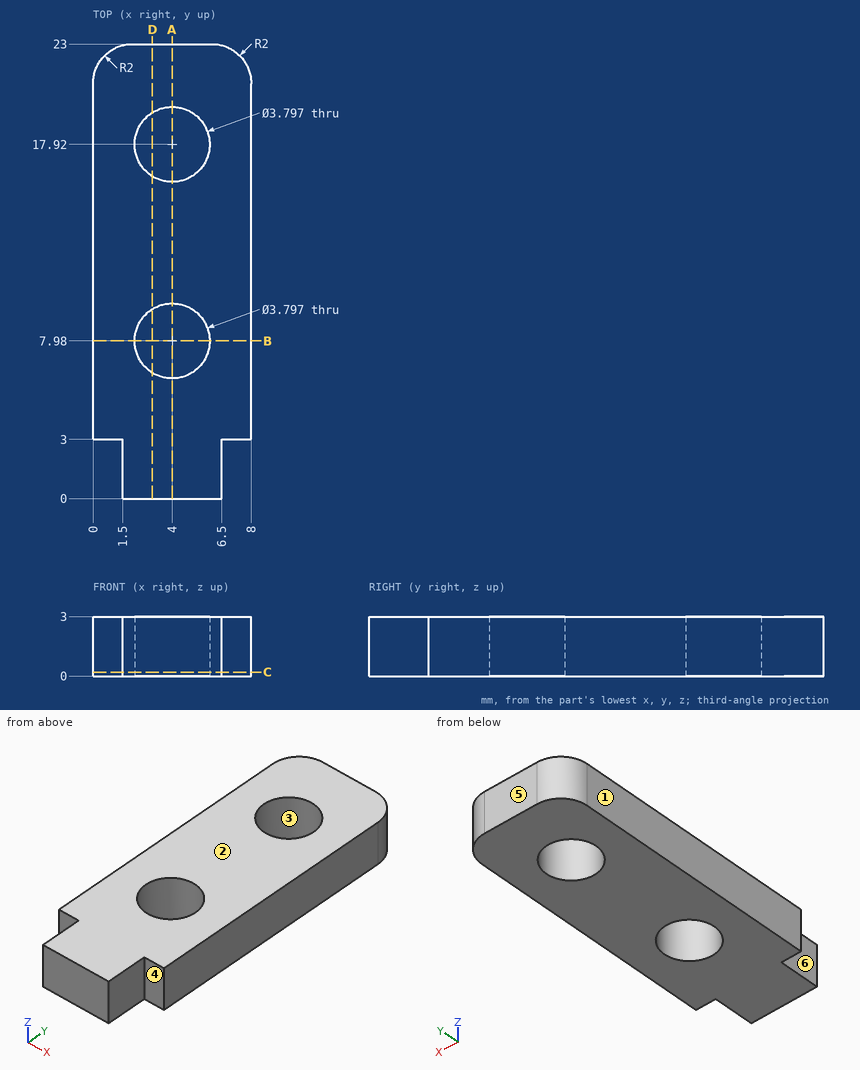
Here's the drawing with two shaded views (mm, measured from the low corner). I have some questions. A direction names the side the tool comes from. Give positions to 0.01 mm unless a question says otherwise; leave off trailing zeros. Order: outer loops, then holes, each group sorted by start corner. A loop starts at its lowest first (then second) coordinate and runs counter-clockwise, first axis right, second up. Notation, with made-up numbers: (21, -10.75) -> (70, -10.75) arc R28 cw to (70, 10.25) -> close; hole circle Ø9 at (4.25, 49). An arc over 180 degrees is marked (long way). One line per item, written item: value. Start each with the question number.
1. For the marked faces 4, 5 and 6, which set-ups out of +Z, -Z, +X, -X, +Y, -Y let a thin tool reach every point of the face, with its end or its side?
2. We'd pull the mould along X, two halves only. Please class the marked faces 1, 2 and 3: released by +X, released by -X, zero draft, split by the parting line, or undercut.
3. I need wall thicknesses on probe 1 along Y at (x, z) = (4, 1.25); probe 2 along Y at (x, z) = (3.25, 1.35) (1 decimal); probe 3 along X at (y, z) = (19, 2.5). Which ranges of each line are inside material? Lowest first, please. Write a range as from..to.
4. Imagine slicing it at A-A, the plane x = 4. List the corners of the cut face in (y, z) for me, plus the area to 3 significant figures.
5. Imagine slicing it at D-D, the plane x = 3. List the corners of the cut face in (y, z) for me.
6. Imagine slicing it at B-B, the plane y = 7.98. List the corners of the cut face in (x, z) for me.
7. Will these pins go through, and if not, where does the flat tip stop? pin 1 Ø0.8 at (x, z) = (1, 2) entering from -Y; pin 2 Ø1.5 at (y, z) = (1.5, 1) entering from -X.
8. Imagine slicing it at C-C, the plane z = 0.2. List the corners of the cut face in (x, y) for me.
Values follow:
1. face 4: +Z, -Z, +X, -Y
1. face 5: +Z, -Z, +X, -X, +Y
1. face 6: +Z, -Z, -X, -Y
2. face 1: released by -X
2. face 2: zero draft
2. face 3: undercut
3. probe 1: y = 0..6.08, 9.88..16.02, 19.82..23
3. probe 2: y = 0..6.2, 9.7..16.2, 19.7..23
3. probe 3: x = 0..2.44, 5.56..8
4. outline: (0, 0) -> (6.08, 0) -> (6.08, 3) -> (0, 3) -> close; (9.88, 0) -> (16.02, 0) -> (16.02, 3) -> (9.88, 3) -> close; (19.82, 0) -> (23, 0) -> (23, 3) -> (19.82, 3) -> close
4. area: 46.2 mm2
5. outline: (0, 0) -> (6.37, 0) -> (6.37, 3) -> (0, 3) -> close; (9.59, 0) -> (16.31, 0) -> (16.31, 3) -> (9.59, 3) -> close; (19.53, 0) -> (23, 0) -> (23, 3) -> (19.53, 3) -> close
6. outline: (0, 0) -> (2.1, 0) -> (2.1, 3) -> (0, 3) -> close; (5.9, 0) -> (8, 0) -> (8, 3) -> (5.9, 3) -> close
7. pin 1: stops at y = 3
7. pin 2: stops at x = 1.5
8. outline: (0, 3) -> (1.5, 3) -> (1.5, 0) -> (6.5, 0) -> (6.5, 3) -> (8, 3) -> (8, 21) arc R2 ccw to (6, 23) -> (2, 23) arc R2 ccw to (0, 21) -> close; hole circle Ø3.8 at (4, 7.98); hole circle Ø3.8 at (4, 17.92)
